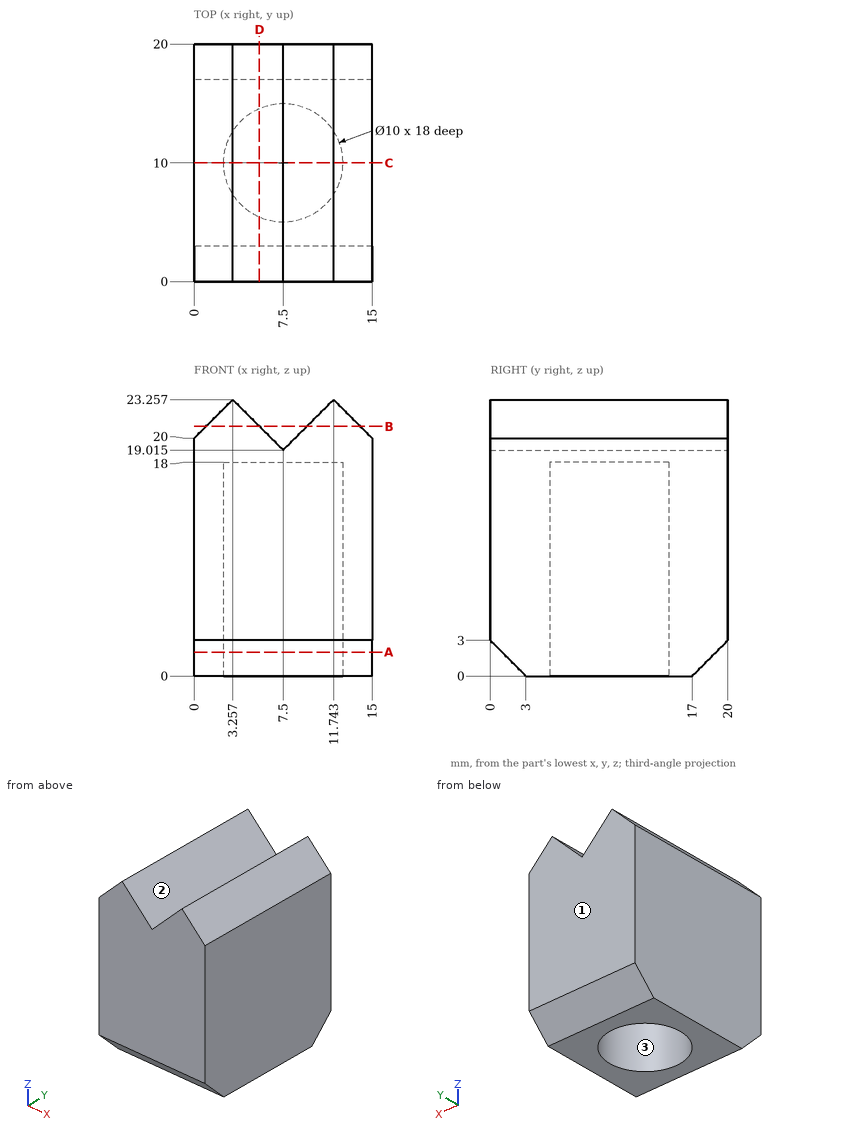
Job drawing, mm, ordinate dimensions from the low corner. One solid piece. Round coordinates to 2 decimals unless told otherwise and drop trailing zeros. Order: outer loops, then holes, each group sorted by start corner. A loop starts at its lowest first (then second) coordinate and runs counter-clockwise, first axis right, second up. Notation, with made-up numbers: M -8.5,38.25 L 42.5,38.25 A19 cw 42.5,74.25 Z; hole C 56,41.5 d3. An arc over 180 degrees is marked long. Write each question's results on one line, items separated by ' | '. Start each with the question number.
(1) Drop flat-ended pins along their axis: pin 1 (8 mm diameter, centred on x = 9, y = 6.5, fed in from -Z); pin 2 (9 mm diameter, centred on x = 7.5, y = 10, fed in from -Z); pin 3 (3 mm diameter, centred on x = 5.5, y = 3.5, fed in from +Z) (1 decimal). Give the stop position or say it passes through.
(2) Two-plate mould, pull along Y, no slides. Class the marked faces 1, 2 and 3: pulls with the +Y half, pulls with the -Y half, needs draft (parallel to the pull), parting line crosses it, or undercut.
(3) Saw through at A-A, the plane z = 2. Give the cut face in (x, y).
(4) Saw through at B-B, the plane z = 21. Give the cut face in (x, y) (1 decimal), then the cut area to 3 significant figures.
(5) Saw through at C-C, the plane y = 10. Give the cut face in (x, z) (1 decimal), then the cut area to 3 significant figures.
(6) Probe probe 1 along Y at (x, z) = (7.5, 13.75); probe 2 along X at (y, z) = (10.25, 1.75); probe 3 along Y at (x, z) = (9, 13.5). List the from-to ranges inside material, lowest first. Write a range as from..to.
(7) Saw through at D-D, the plane x = 5.5. Give the cut face in (y, z) (1 decimal), then the cut area to 3 significant figures.
Established:
1) pin 1: stops at z = 0 | pin 2: stops at z = 18 | pin 3: stops at z = 22.5
2) face 1: pulls with the +Y half | face 2: needs draft | face 3: undercut
3) outline: M 0,1 L 15,1 L 15,19 L 0,19 Z; hole C 7.5,10 d10
4) outline: M 1,0 L 5.5,0 L 5.5,20 L 1,20 Z; M 9.5,0 L 14,0 L 14,20 L 9.5,20 Z | area: 181 mm^2
5) outline: M 0,0 L 2.5,0 L 2.5,18 L 12.5,18 L 12.5,0 L 15,0 L 15,20 L 11.7,23.3 L 7.5,19 L 3.3,23.3 L 0,20 Z | area: 140 mm^2
6) probe 1: y = 0..5, 15..20 | probe 2: x = 0..2.51, 12.49..15 | probe 3: y = 0..5.23, 14.77..20
7) outline: M 0,3 L 3,0 L 5.4,0 L 5.4,18 L 14.6,18 L 14.6,0 L 17,0 L 20,3 L 20,21 L 0,21 Z | area: 246 mm^2
